Could you check a few things on this drawing? It's one solid part, dimensions in mm from its lowest x, y, z. Give positions to 0.01 mm unless a question says otherwise; leave off trailing zeros. Order: outer loops, then holes, each group sorted by start corner. A loop starts at its lowest first (then second) coordinate and runs counter-clockwise, first axis right, second up.
(1) Imagine slicing it at A-A, the plane y = 8.25. Write out the boundary of the cut face in (x, z) (1 decimal).
(2) Imagine slicing it at C-C, the plane z = 1.3. Write out the boundary of the cut face in (x, y) (1 decimal).
(3) Will this pin go through, and if not, where does the flat tip stop? pin 1 (1 mm diameter, centred on y = 5, z = 2, fed in from +X).
(4) Imagine slicing it at D-D, the plane x = 11.5. Write out the boundary of the cut face in (y, z).
(5) If I drill on probe 1 along X at (y, z) = (6.44, 0.75); probe 2 along Y at (x, z) = (6.44, 1.55); probe 3 along X at (y, z) = (11.5, 1.85) (1 decimal), over which ranges is the centre line in solid material (lowest first)?
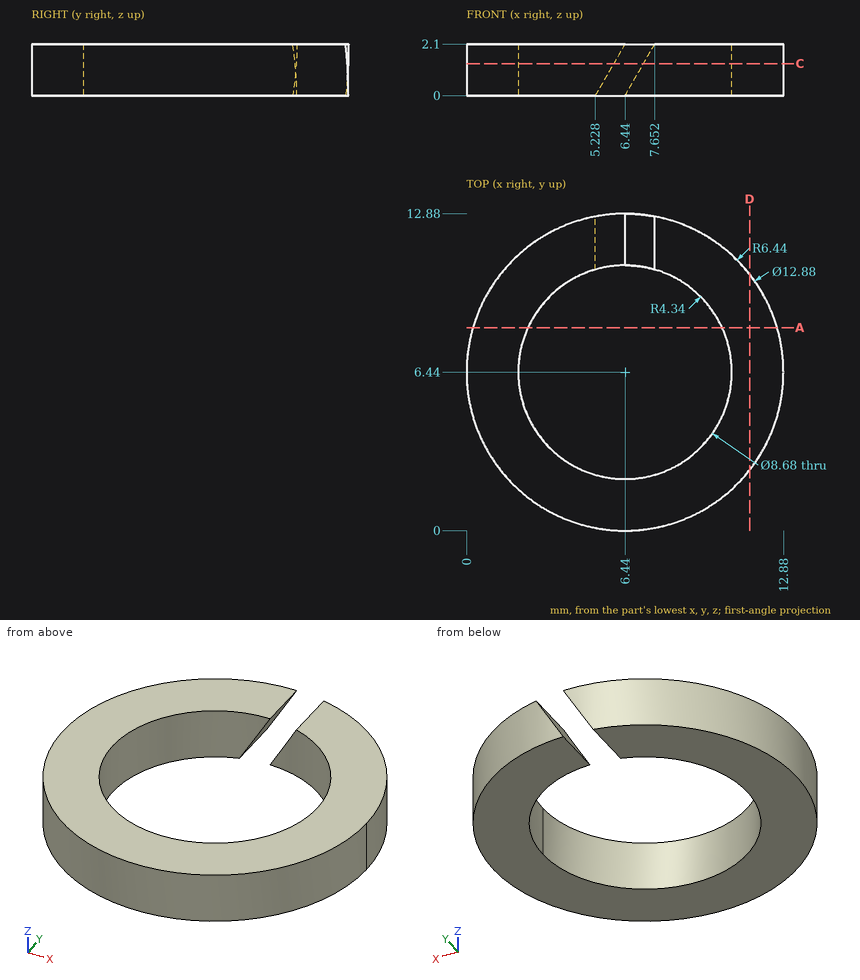
Answer block:
1. outline: (0.3, 0) - (2.5, 0) - (2.5, 2.1) - (0.3, 2.1) - close; (10.4, 0) - (12.6, 0) - (12.6, 2.1) - (10.4, 2.1) - close
2. outline: (6, 10.8) - (6, 12.9) arc R6.4 ccw (long way) to (7.2, 12.8) - (7.2, 10.7) arc R4.3 cw (long way) to start
3. pin 1: stops at x = 12.81
4. outline: (2.46, 0) - (10.42, 0) - (10.42, 2.1) - (2.46, 2.1) - close
5. probe 1: x = 0 to 2.1, 10.78 to 12.88
5. probe 2: y = 0 to 2.1
5. probe 3: x = 2.5 to 6.3, 7.5 to 10.4
